from build123d import *

# Parameters (mm, degrees)
F1_DEPTH = 25
F2_R     = 2
F3_R     = 4
F4_R     = 5
F5_DEPTH = 0.01


with BuildPart() as f1:
    # F0 (on Top) → F1 (new body, symmetric)
    with BuildSketch(Plane.XY):
        Polygon((140, 0), (0, 0), (-140, 0), (-140, -30), (-120, -30), (-120, -28), (-138, -28), (-138, -2), (0, -2), (138, -2), (138, -28), (120, -28), (120, -30), (140, -30), align=None)
    extrude(amount=F1_DEPTH, both=True)

    # F2
    f2_edges = [f1.edges().sort_by_distance(p)[0] for p in [
        (-138, -28, 0),
        (-138, -2, 0),
        (138, -28, 0),
        (138, -2, 0),
    ]]
    fillet(f2_edges, radius=F2_R)

    # F3
    f3_edges = [f1.edges().sort_by_distance(p)[0] for p in [
        (-140, -30, 0),
        (-140, 0, 0),
        (140, -30, 0),
        (140, 0, 0),
    ]]
    fillet(f3_edges, radius=F3_R)

    # F4 (on face) → F5 (cut)
    with BuildSketch(Plane.XZ.offset(2)):
        with Locations((0, 18)):
            Circle(F4_R)
    extrude(amount=-F5_DEPTH, mode=Mode.SUBTRACT)


solid = f1.part
Geometry check sheet. Reference: the model listing, model coordinates, mm. A direction names the side the tool comes from. Round coordinates to 2 decimals unless told otherwise and drop trailing zeros. Loops run counter-clockwise (first coordinate to the right, second up) from the corner with the lowest first, then second, coordinate; pieces in that order, holes last. Notation, with made-up numbers: (-1, -3) - (11, -3) arc R28 cw to (11, 15) - close; hole circle Ø10 at (40.5, -34.75). An arc over 180 degrees is marked (long way). Answer as CSV lines item,"result".
(1) Material ranges on line 1 along X through (y, z) = (-16.5, -17); line 2 along Y through (x, z) = (123, -11.5); line 3 along Y through (x, z) = (48.5, 12), recorded low to high.
Output values:
line 1,"x = -140 to -138, 138 to 140"
line 2,"y = -30 to -28, -2 to 0"
line 3,"y = -2 to 0"
(2) Cross-section at B-B, the plane y = -19.75. Enter the section's corners in (x, z).
Output values:
outline,"(-140, -25) - (-138, -25) - (-138, 25) - (-140, 25) - close; (138, -25) - (140, -25) - (140, 25) - (138, 25) - close"
(3) Depth check by flat-ended pin: pin 1 Ø15 at (x, z) = (26, -10) entering from -Y; pin 2 Ø1 at (y, z) = (-28.5, 4.5) entering from +X; pin 3 Ø1 at (y, z) = (-29.5, 11.5) entering from -X. Enter the tip coordinate at first touch or a pass-through.
Output values:
pin 1,"stops at y = -2"
pin 2,"stops at x = 139.46"
pin 3,"stops at x = -138.65"
(4) Release check for a two-part mould opening along Y. For faces 1 (the face through (128, -28, 0)), 2 (the face through (-128, -28, 0)), 3 (the face through (-140, -15, 0)), 4 (the face through (128, -30, 0)) record: released by +Y, released by -Y, zero draft, split by the parting line, or undercut.
Output values:
face 1,"undercut"
face 2,"undercut"
face 3,"zero draft"
face 4,"released by -Y"
(5) Set-up check for faces 5 (the face through (140, -15, 0)), 6 (the face through (0, -1.99, 18)), 7 (the face through (138, -15, 0)): record each of +Z, -Z, +X, -X, +Y, -Y from which the full face is reachable in a straight line by a thin tool's end or side.
Output values:
face 5,"+Z, -Z, +X, +Y, -Y"
face 6,"+Z, -Z, -Y"
face 7,"+Z, -Z"
(6) Cross-section at D-D, the plane z = 1.5. Enter the section's corners in (x, y), and give its area (3 significant figures).
Output values:
outline,"(-140, -26) arc R4 ccw to (-136, -30) - (-120, -30) - (-120, -28) - (-136, -28) arc R2 cw to (-138, -26) - (-138, -4) arc R2 cw to (-136, -2) - (136, -2) arc R2 cw to (138, -4) - (138, -26) arc R2 cw to (136, -28) - (120, -28) - (120, -30) - (136, -30) arc R4 ccw to (140, -26) - (140, -4) arc R4 ccw to (136, 0) - (-136, 0) arc R4 ccw to (-140, -4) - close"
area,"734 mm²"
